Here's how the part is built. I have some questions about the finished solid (model axes, mm). A direction names the side the tool comes from. Coordinates: 2 decimals unless noted, no trailing zeros. Write each loop counter-clockwise with the first axis right and the second up, starting at its lowest first coordinate (ties: lowest second). Pieces come first, ordered by that corner, then holes. Notation, with made-up numbers: (50, 25) -> (76, 25) arc R19 ccw to (76, 47) -> close; hole circle Ø4 at (13, 43). An arc over 180 degrees is marked (long way). Use a Markdown table: item, result. Add a question column.
Item 1: If I drill on line 1 along X through (y, z) = (28.5, 52.5); line 2 along Z through (x, y) = (-4.5, -2); line 3 along Z through (x, y) = (-56, -7.5), over which ranges is the centre line in solid material (lowest first)? Write a range as from..to.
Item 2: Imagine slicing it at A-A, the plane y = 25. Write out the boundary of the cut face in (x, z).
Item 3: Imagine slicing it at B-B, the plane x = 16.5. Write out the boundary of the cut face in (y, z), and give its area (3 significant figures).
Item 4: Will these pins go through, and if not, where does the flat tip stop? pin 1 Ø9.5 at (x, y) = (1.5, -15.5) entering from +Z; pin 2 Ø12 at (y, z) = (24.5, 43.5) entering from +X; pin 3 Ø2 at (y, z) = (-11.5, 42) entering from +X.
Item 5: Imagine slicing it at C-C, the plane x = -19.5. Write out the boundary of the cut face in (y, z).
Item 6: On a 3-axis mill with a long thin cutter (end or side, diameter ignored), from which of +Z, -Z, +X, -X, +Y, -Y can I reach the whole of each face in a straight line? I mean faces 1 (the flat face through (-19.78, 34.73, 59.79)), 2 (the flat face through (-19.78, -43.4, 59.79)), 3 (the flat face through (-17.316, -5, 60)), 4 (the flat face through (24.494, -5, 20)), 5 (the flat face through (22.029, -4.847, 2.535)). Say none if no direction works.
```python
from build123d import *

# Parameters (mm, degrees)
F0_W     = 83.6216490716
F0_H     = 83.1985995173
F1_DEPTH = 40
F2_W     = 41.8108245358
F2_H     = 83.1985995173
F3_DEPTH = 40
F4_SIZE  = 5


with BuildPart() as f1:
    # F0 (on Top) → F1 (new body)
    with BuildSketch(Plane.XY):
        with Locations((-17.3164242879, -4.335001111)):
            Rectangle(F0_W, F0_H)
    extrude(amount=F1_DEPTH)

    # F2 (on face) → F3 (join)
    with BuildSketch(Plane.XY.offset(40)):
        with Locations((-38.2218365557, -4.335001111)):
            Rectangle(F2_W, F2_H)
    extrude(amount=F3_DEPTH)

    # F4
    f4_edges = [f1.edges().sort_by_distance(p)[0] for p in [
        (-17.316424, -4.335001, 80),
        (-38.221837, 37.264299, 80),
        (-59.127249, -4.335001, 80),
        (-38.221837, -45.934301, 80),
        (-59.127249, -45.934301, 40),
        (-17.316424, -45.934301, 60),
        (3.588988, -45.934301, 40),
        (24.4944, -45.934301, 20),
        (-17.316424, -45.934301, 0),
        (3.588988, 37.264299, 40),
        (24.4944, -4.335001, 40),
        (-17.316424, -4.335001, 40),
        (-17.316424, 37.264299, 60),
        (24.4944, 37.264299, 20),
        (24.4944, -4.335001, 0),
        (-59.127249, 37.264299, 40),
        (-17.316424, 37.264299, 0),
    ]]
    chamfer(f4_edges, length=F4_SIZE)


solid = f1.part
```
Ans:
| question | item | result |
|---|---|---|
| 1 | line 1 | x = -59.13..-17.32 |
| 1 | line 2 | z = 0..40 |
| 1 | line 3 | z = 0..78.13 |
| 2 | outline | (-59.13, 0) -> (19.49, 0) -> (24.49, 5) -> (24.49, 35) -> (19.49, 40) -> (-12.32, 40) -> (-17.32, 45) -> (-17.32, 75) -> (-22.32, 80) -> (-54.13, 80) -> (-59.13, 75) -> close |
| 3 | outline | (-45.93, 5) -> (-40.93, 0) -> (32.26, 0) -> (37.26, 5) -> (37.26, 35) -> (32.26, 40) -> (-40.93, 40) -> (-45.93, 35) -> close |
| 3 | area | 3,280 mm^2 |
| 4 | pin 1 | stops at z = 40 |
| 4 | pin 2 | stops at x = 21.99 |
| 4 | pin 3 | stops at x = -13.32 |
| 5 | outline | (-45.93, 5) -> (-40.93, 0) -> (32.26, 0) -> (37.26, 5) -> (37.26, 42.18) -> (34.45, 45) -> (34.45, 75) -> (32.26, 77.18) -> (-40.93, 77.18) -> (-43.12, 75) -> (-43.12, 45) -> (-45.93, 42.18) -> close |
| 6 | face 1 | +Z, +X, +Y |
| 6 | face 2 | +Z, +X, -Y |
| 6 | face 3 | +Z, +X, +Y, -Y |
| 6 | face 4 | +Z, -Z, +X, +Y, -Y |
| 6 | face 5 | -Z, +X, +Y, -Y |
